Autodesk Inventor part; units mm, degrees
ref_plane "YZ Plane" through (0, 0, 0) normal (1, 0, 0) x (0, 1, 0)
ref_plane "XZ Plane" through (0, 0, 0) normal (0, 1, 0) x (-1, 0, 0)
ref_plane "XY Plane" through (0, 0, 0) normal (0, 0, 1) x (1, 0, 0)
sketch "Sketch1" plane through (0, 0, 0) normal (1, 0, 0) x (0, 1, 0)
  circle A0 centre (0, 0) radius 4.7625
  dimension "d0" = 9.525
extrude "Extrusion1" add sketch "Sketch1" along normal blind 3.175
sketch "Sketch2" plane through (3.175, 0, 0) normal (1, 0, 0) x (0, 0, -1)
  circle A0 centre (0, 0) radius 4.7625
  circle A1 centre (0, 0) radius 5.334
  dimension "d4" = 10.668
extrude "Extrusion2" add sketch "Sketch2" along normal blind 0.889 contours A0 | A1
sketch "Sketch3" plane through (4.064, 0, 0) normal (1, 0, 0) x (0, 0, -1)
  circle A0 centre (0, 0) radius 5.334
hole "Hole1" at (4.064, 0, 0) direction (-1, 0, 0) diameter 4.826 end through all
properties part number "Clutch Bearing" material "Brass, Soft Yellow"
CAD build for the part. Positions are in the model's coordinates, mm. A direction names the side the tool comes from. Coordinates: 2 decimals unless noted, no trailing zeros. Loops run counter-clockwise (first coordinate to the right, second up) from the corner with the lowest first, then second, coordinate; pieces in that order, holes last. Notation, with made-up numbers: (31.5, 4.5) -> (60.5, 4.5) arc R17 cw to (60.5, 37.5) -> close; hole circle Ø3 at (47.25, -33). An arc over 180 degrees is marked (long way). One line per item, written item: value.
1. Slice it at A-A on y = 0. Write the cut outline in (x, z) (1 decimal).
Answers:
outline: (0, -4.8) -> (3.2, -4.8) -> (3.2, -5.3) -> (4.1, -5.3) -> (4.1, -2.4) -> (0, -2.4) -> close; (0, 2.4) -> (4.1, 2.4) -> (4.1, 5.3) -> (3.2, 5.3) -> (3.2, 4.8) -> (0, 4.8) -> close
2. Drill centre lines: line 1 (Z direction, x = 3.1, y = 0); line 2 (Y direction, x = 1.9, z = -1); line 3 (X direction, y = -4.25, z = 2.5) (3 decimals). Where is each one in solid material? Low to high. Write a range as [from, to].
Answers:
line 1: z = [-4.76, -2.41], [2.41, 4.76]
line 2: y = [-4.66, -2.2], [2.2, 4.66]
line 3: x = [3.175, 4.064]
3. Flat gauge pins, fed straight in: P1, Ø3, axis at y = -1.5, z = -1.5, coming from the -X side; P2, Ø1, axis at x = 1, z = -2.5, coming from the -Y side. Where does each tip first touch, or does it go through?
Answers:
P1: stops at x = 0
P2: stops at y = -4.32
4. Slice it at C-C on x = 2.75. Write the cut outline in (y, z) (1 decimal), and give its area (3 significant figures).
Answers:
outline: circle Ø9.5 at (0, 0); hole circle Ø4.8 at (0, 0)
area: 53.0 mm^2
5. Pull direction Z, two halves, no side cores. Call faces 1 (the face through (2.004, 1.468, 1.915)), 2 (the face through (1.57, -3.78, 2.9)), 3 (the face through (4.064, 1.3, -2.3)): pulls with the +Z half, pulls with the -Z half, needs draft (parallel to the pull), parting line crosses it, or undercut.
Answers:
face 1: undercut
face 2: parting line crosses it
face 3: needs draft
6. Slice it at D-D on z = 4.5. Write the cut outline in (x, y) (3 decimals).
Answers:
outline: (0, -1.559) -> (3.175, -1.559) -> (3.175, -2.864) -> (4.064, -2.864) -> (4.064, 2.864) -> (3.175, 2.864) -> (3.175, 1.559) -> (0, 1.559) -> close
7. Which spindle directions (+Z, -Z, +X, -X, +Y, -Y) get a long thin tool onto all of the face, cutting with end or side? Do faces 4 (the face through (3.613, 4.732, -2.461)), 5 (the face through (3.175, 3, 4)). Say none if no direction does.
Answers:
face 4: +X, -X
face 5: -X
